Could you check a few things on this model? Use its own coordinates, in mm. Give positions to 0.01 mm unless a question says otherwise; leave off trailing zeros. Order: outer loops, then holes, each group sorted by start corner. A loop starts at its lowest first (then second) coordinate and runs counter-clockwise, first axis right, second up. Notation, with made-up numbers: M 14,-1 L 57,-1 A36 ccw 57,34 Z; hole C 4,7.25 d8. An arc over 180 degrees is marked long. Use a Markdown table: item, result. Add a question column.
Item 1: If we mould it in two halves opening along Y, with no side actions, what happens to faces 1 (the face through (-57, 88, 3)), 2 (the face through (-37.8, 63.7, 1.5)), 3 (the face through (-8.227, 104.203, 1.479))? For each: released by +Y, released by -Y, zero draft, split by the parting line, or undercut.
Item 2: If I drill on L1, parallel to Y at x = -20.5, z = 1; L2, parallel to Y at x = -74, z = 0.75; L3, parallel to X at y = 103, z = 0.7, over which ranges is the centre line in solid material (lowest first)? Write a range as from..to.
Item 3: Suppose I cut it at B-B on z = 1.2. Count the separate pieces of the cut face and the enclosed holes in it, plus the area to 3 significant figures.
Item 4: Suppose I cut it at A-A on x = -20.5. Write out the boundary of the cut face in (y, z).
from build123d import *

# Parameters (mm, degrees)
MODEL_R                 = 1.5
SALIENTE_EXTRUIR1_DEPTH = 3


with BuildPart() as part:
    # Model → Saliente-Extruir1 (new body)
    with BuildSketch(Plane.XY):
        with BuildLine():
            Line((-105.943383637, 101.056539338), (-105.943383637, 65.056539338))
            ThreePointArc((-105.943383637, 65.056539338), (-104.625364152, 61.874558823), (-101.443383637, 60.556539338))
            Line((-101.443383637, 60.556539338), (-11.443383637, 60.556539338))
            ThreePointArc((-11.443383637, 60.556539338), (-8.261403122, 61.874558823), (-6.943383637, 65.056539338))
            Line((-6.943383637, 65.056539338), (-6.943383637, 101.056539338))
            ThreePointArc((-6.943383637, 101.056539338), (-8.261403122, 104.238519853), (-11.443383637, 105.556539338))
            Line((-11.443383637, 105.556539338), (-101.443383637, 105.556539338))
            ThreePointArc((-101.443383637, 105.556539338), (-104.625364152, 104.238519853), (-105.943383637, 101.056539338))
        make_face()
        with Locations((-101.443383637, 101.056539338)):
            Circle(MODEL_R, mode=Mode.SUBTRACT)
        with Locations((-92.443383637, 101.056539338)):
            Circle(MODEL_R, mode=Mode.SUBTRACT)
        with Locations((-83.443383637, 101.056539338)):
            Circle(MODEL_R, mode=Mode.SUBTRACT)
        with Locations((-74.443383637, 101.056539338)):
            Circle(MODEL_R, mode=Mode.SUBTRACT)
        with Locations((-65.443383637, 101.056539338)):
            Circle(MODEL_R, mode=Mode.SUBTRACT)
        with Locations((-56.443383637, 101.056539338)):
            Circle(MODEL_R, mode=Mode.SUBTRACT)
        with Locations((-47.443383637, 101.056539338)):
            Circle(MODEL_R, mode=Mode.SUBTRACT)
        with Locations((-20.443383637, 101.056539338)):
            Circle(MODEL_R, mode=Mode.SUBTRACT)
        with Locations((-101.443383637, 92.056539338)):
            Circle(MODEL_R, mode=Mode.SUBTRACT)
        with Locations((-92.443383637, 92.056539338)):
            Circle(MODEL_R, mode=Mode.SUBTRACT)
        with Locations((-83.443383637, 92.056539338)):
            Circle(MODEL_R, mode=Mode.SUBTRACT)
        with Locations((-74.443383637, 92.056539338)):
            Circle(MODEL_R, mode=Mode.SUBTRACT)
        with Locations((-65.443383637, 92.056539338)):
            Circle(MODEL_R, mode=Mode.SUBTRACT)
        with Locations((-56.443383637, 92.056539338)):
            Circle(MODEL_R, mode=Mode.SUBTRACT)
        with Locations((-47.443383637, 92.056539338)):
            Circle(MODEL_R, mode=Mode.SUBTRACT)
        with Locations((-20.443383637, 92.056539338)):
            Circle(MODEL_R, mode=Mode.SUBTRACT)
        with Locations((-101.443383637, 83.056539338)):
            Circle(MODEL_R, mode=Mode.SUBTRACT)
        with Locations((-92.443383637, 83.056539338)):
            Circle(MODEL_R, mode=Mode.SUBTRACT)
        with Locations((-83.443383637, 83.056539338)):
            Circle(MODEL_R, mode=Mode.SUBTRACT)
        with Locations((-74.443383637, 83.056539338)):
            Circle(MODEL_R, mode=Mode.SUBTRACT)
        with Locations((-65.443383637, 83.056539338)):
            Circle(MODEL_R, mode=Mode.SUBTRACT)
        with Locations((-56.443383637, 83.056539338)):
            Circle(MODEL_R, mode=Mode.SUBTRACT)
        with Locations((-47.443383637, 83.056539338)):
            Circle(MODEL_R, mode=Mode.SUBTRACT)
        with Locations((-20.443383637, 83.056539338)):
            Circle(MODEL_R, mode=Mode.SUBTRACT)
        with Locations((-101.443383637, 65.056539338)):
            Circle(MODEL_R, mode=Mode.SUBTRACT)
        with Locations((-92.443383637, 65.056539338)):
            Circle(MODEL_R, mode=Mode.SUBTRACT)
        with Locations((-83.443383637, 65.056539338)):
            Circle(MODEL_R, mode=Mode.SUBTRACT)
        with Locations((-74.443383637, 65.056539338)):
            Circle(MODEL_R, mode=Mode.SUBTRACT)
        with Locations((-65.443383637, 65.056539338)):
            Circle(MODEL_R, mode=Mode.SUBTRACT)
        with Locations((-56.443383637, 65.056539338)):
            Circle(MODEL_R, mode=Mode.SUBTRACT)
        with Locations((-47.443383637, 65.056539338)):
            Circle(MODEL_R, mode=Mode.SUBTRACT)
        with Locations((-20.443383637, 65.056539338)):
            Circle(MODEL_R, mode=Mode.SUBTRACT)
        with Locations((-11.443383637, 101.056539338)):
            Circle(MODEL_R, mode=Mode.SUBTRACT)
        with Locations((-11.443383637, 92.056539338)):
            Circle(MODEL_R, mode=Mode.SUBTRACT)
        with Locations((-11.443383637, 83.056539338)):
            Circle(MODEL_R, mode=Mode.SUBTRACT)
        with Locations((-11.443383637, 65.056539338)):
            Circle(MODEL_R, mode=Mode.SUBTRACT)
        with Locations((-101.443383637, 74.056539338)):
            Circle(MODEL_R, mode=Mode.SUBTRACT)
        with Locations((-92.443383637, 74.056539338)):
            Circle(MODEL_R, mode=Mode.SUBTRACT)
        with Locations((-83.443383637, 74.056539338)):
            Circle(MODEL_R, mode=Mode.SUBTRACT)
        with Locations((-74.443383637, 74.056539338)):
            Circle(MODEL_R, mode=Mode.SUBTRACT)
        with Locations((-65.443383637, 74.056539338)):
            Circle(MODEL_R, mode=Mode.SUBTRACT)
        with Locations((-56.443383637, 74.056539338)):
            Circle(MODEL_R, mode=Mode.SUBTRACT)
        with Locations((-47.443383637, 74.056539338)):
            Circle(MODEL_R, mode=Mode.SUBTRACT)
        with Locations((-20.443383637, 74.056539338)):
            Circle(MODEL_R, mode=Mode.SUBTRACT)
        with Locations((-11.443383637, 74.056539338)):
            Circle(MODEL_R, mode=Mode.SUBTRACT)
        with Locations((-38.443383637, 101.056539338)):
            Circle(MODEL_R, mode=Mode.SUBTRACT)
        with Locations((-29.443383637, 101.056539338)):
            Circle(MODEL_R, mode=Mode.SUBTRACT)
        with Locations((-38.443383637, 92.056539338)):
            Circle(MODEL_R, mode=Mode.SUBTRACT)
        with Locations((-29.443383637, 92.056539338)):
            Circle(MODEL_R, mode=Mode.SUBTRACT)
        with Locations((-38.443383637, 83.056539338)):
            Circle(MODEL_R, mode=Mode.SUBTRACT)
        with Locations((-29.443383637, 83.056539338)):
            Circle(MODEL_R, mode=Mode.SUBTRACT)
        with Locations((-38.443383637, 65.056539338)):
            Circle(MODEL_R, mode=Mode.SUBTRACT)
        with Locations((-29.443383637, 65.056539338)):
            Circle(MODEL_R, mode=Mode.SUBTRACT)
        with Locations((-38.443383637, 74.056539338)):
            Circle(MODEL_R, mode=Mode.SUBTRACT)
        with Locations((-29.443383637, 74.056539338)):
            Circle(MODEL_R, mode=Mode.SUBTRACT)
    extrude(amount=SALIENTE_EXTRUIR1_DEPTH)


solid = part.part
Findings below:
| question | item | result |
|---|---|---|
| 1 | face 1 | zero draft |
| 1 | face 2 | undercut |
| 1 | face 3 | released by +Y |
| 2 | L1 | y = 60.56..63.56, 66.56..72.56, 75.56..81.56, 84.56..90.56, 93.56..99.56, 102.56..105.56 |
| 2 | L2 | y = 60.56..63.62, 66.49..72.62, 75.49..81.62, 84.49..90.62, 93.49..99.62, 102.49..105.56 |
| 2 | L3 | x = -105.5..-7.38 |
| 3 | separate pieces | 1 |
| 3 | enclosed holes | 55 |
| 3 | area | 4,050 mm^2 |
| 4 | outline | M 60.56,0 L 63.56,0 L 63.56,3 L 60.56,3 Z; M 66.56,0 L 72.56,0 L 72.56,3 L 66.56,3 Z; M 75.56,0 L 81.56,0 L 81.56,3 L 75.56,3 Z; M 84.56,0 L 90.56,0 L 90.56,3 L 84.56,3 Z; M 93.56,0 L 99.56,0 L 99.56,3 L 93.56,3 Z; M 102.56,0 L 105.56,0 L 105.56,3 L 102.56,3 Z |
